from build123d import *

# Parameters (mm, degrees)
F0_R     = 7.1
F0_R_2   = 5.5
F1_DEPTH = 40
F2_START = 19.8
F0_R_3   = 5.1
F2_DEPTH = 0.4
F3_SIZE  = 0.39999
F4_SIZE  = 0.4


# Not quite as in the source:
# - a fillet or chamfer is up to 0.001 mm smaller than in the source, because OpenCascade refuses the exact size


with BuildPart() as f1:
    # F0 (on Top) → F1 (new body)
    with BuildSketch(Plane.XY):
        Circle(F0_R)
        Circle(F0_R_2, mode=Mode.SUBTRACT)
    extrude(amount=F1_DEPTH)

    # F0 (on Top) → F2 (join)
    with BuildSketch(Plane.XY.offset(F2_START)):
        Circle(F0_R_2)
        Circle(F0_R_3, mode=Mode.SUBTRACT)
    extrude(amount=F2_DEPTH)

    # F3 (size 0.4 in the source; OpenCascade refuses exactly that, so slightly less here)
    f3_edges = [f1.edges().sort_by_distance(p)[0] for p in [
        (-5.5, 0, 19.8),
        (-5.5, 0, 20.2),
    ]]
    chamfer(f3_edges, length=F3_SIZE)

    # F4
    f4_edges = [f1.edges().sort_by_distance(p)[0] for p in [
        (-5.5, 0, 40),
        (-7.1, 0, 40),
        (-5.5, 0, 0),
        (-7.1, 0, 0),
    ]]
    chamfer(f4_edges, length=F4_SIZE)


solid = f1.part
The model under review builds one solid part; all positions refer to its coordinate system, in mm. Give positions to 0.01 mm unless a question says otherwise; leave off trailing zeros. Order: outer loops, then holes, each group sorted by start corner. A loop starts at its lowest first (then second) coordinate and runs counter-clockwise, first axis right, second up. Notation, with made-up numbers: (-1, 47) -> (53, 47) arc R21 ccw to (53, 84) -> close; hole circle Ø3 at (15.25, 62.25). An arc over 180 degrees is marked (long way). Write item = value, one per line. Start each with the question number.
(1) Draft analysis for pull direction X (two halves, no side actions). For faces 1 (the cylindrical face through (-1.19, -5.37, 29.97)), 2 (the cylindrical face through (2.4, -4.5, 20)), 3 (the cylindrical face through (-0.92, 7.04, 19.73)), state which applies: +X half, -X half, draft (parallel to the pull), parting line (faces both ways), or undercut.
(2) Take a section at C-C (z = 25.5). Write out the cut boundary in (x, y), plus the area to 3 significant figures.
(3) For L1, parallel to Y at x = 0, z = 20; L2, parallel to Y at x = 0, z = 35.25; L3, parallel to X at y = -3, z = 34.5, list the stretches that pass through material, from the lowest coordinate up. Write a range as from..to.
(4) For pin 1 Ø8 at (y, z) = (-3, 20.5) entering from +X; pin 2 Ø6 at (x, z) = (-4, 13.5) entering from -Y; pin 3 Ø1 at (y, z) = (5, 12.5) entering from -X, all flat-tipped, find the tip position at first contact; note any pin that passes through.
Returned:
q1.face_1 = undercut
q1.face_2 = undercut
q1.face_3 = parting line
q2.outline = circle Ø14.2 at (0, 0); hole circle Ø11 at (0, 0)
q2.area = 63.3 mm²
q3.L1 = -7.1..-5.1, 5.1..7.1
q3.L2 = -7.1..-5.5, 5.5..7.1
q3.L3 = -6.44..-4.61, 4.61..6.44
q4.pin_1 = 7.1
q4.pin_2 = -7.03
q4.pin_3 = -5.49
